```python
from build123d import *

# Parameters (mm, degrees)
BOSS_EXTRUDE1_DEPTH = 32
SKETCH2_R           = 5
CUT_EXTRUDE1_DEPTH  = 32


with BuildPart() as part:
    # Sketch1 → Boss-Extrude1 (new body)
    with BuildSketch(Plane.XY):
        with BuildLine():
            Line((-30, 0), (-13, 0))
            ThreePointArc((-13, 0), (0, -13), (13, 0))
            Line((13, 0), (30, 0))
            Line((30, 0), (30, -20))
            Line((30, -20), (-30, -20))
            Line((-30, -20), (-30, 0))
        make_face()
    extrude(amount=BOSS_EXTRUDE1_DEPTH)

    # Sketch2 → Cut-Extrude1 (cut)
    with BuildSketch(Plane.XZ.offset(20)):
        with Locations(Location((-19, 16, 0), (0, 0, 270))):
            Circle(SKETCH2_R)
        with Locations(Location((19, 16, 0), (0, 0, 270))):
            Circle(SKETCH2_R)
    extrude(amount=-CUT_EXTRUDE1_DEPTH, mode=Mode.SUBTRACT)


solid = part.part
```
Geometry check sheet. Reference: the model listing, model coordinates, mm. Give positions to 0.01 mm unless a question says otherwise; leave off trailing zeros. Write each loop counter-clockwise with the first axis right and the second up, starting at its lowest first coordinate (ties: lowest second). Pieces come first, ordered by that corner, then holes. Notation, with made-up numbers: (31, 12) -> (38, 12) arc R31 cw to (38, 50) -> close; hole circle Ø9 at (40.25, 41.5). An arc over 180 degrees is marked (long way). Use one line per item in the form item = value.
Item 1: Sectioned sample at C-C on z = 16. Enter the section's corners in (x, y), plus the area to 3 significant figures.
Results list:
outline = (-30, -20) -> (-24, -20) -> (-24, 0) -> (-30, 0) -> close; (-14, -20) -> (14, -20) -> (14, 0) -> (13, 0) arc R13 cw to (-13, 0) -> (-14, 0) -> close; (24, -20) -> (30, -20) -> (30, 0) -> (24, 0) -> close
area = 535 mm2
Item 2: Scan lines: line 1 (X direction, y = -14, z = 16); line 2 (X direction, y = -5.25, z = 16); line 3 (X direction, y = -6.25, z = 16). Record each from-to range of solid material in increasing order.
Results list:
line_1 = -30 to -24, -14 to 14, 24 to 30
line_2 = -30 to -24, -14 to -11.89, 11.89 to 14, 24 to 30
line_3 = -30 to -24, -14 to -11.4, 11.4 to 14, 24 to 30
Item 3: Sectioned sample at D-D on y = -5.75. Enter the section's corners in (x, z).
Results list:
outline = (-30, 0) -> (-11.66, 0) -> (-11.66, 32) -> (-30, 32) -> close; (11.66, 0) -> (30, 0) -> (30, 32) -> (11.66, 32) -> close; hole circle Ø10 at (-19, 16); hole circle Ø10 at (19, 16)
Item 4: Mould release check, pull along Z, two halves, no side actions. Record for faces 1 (the flat face through (25, 0, 16)), 2 (the flat face through (0, -14, 0)), 3 (the cylindrical face through (14.12, -10.14, 17.08)), 4 (the flat face through (0, -14, 32)): released by +Z, released by -Z, zero draft, split by the parting line, or undercut.
Results list:
face_1 = zero draft
face_2 = released by -Z
face_3 = undercut
face_4 = released by +Z
Item 5: Depth check by flat-ended pin: pin 1 Ø1.5 at (x, z) = (22.5, 17) entering from -Y. Enter the tip coordinate at first touch or a pass-through.
Results list:
pin_1 = through
Item 6: Sectioned sample at B-B on x = 19. Enter the section's corners in (y, z), plus the area to 3 significant figures.
Results list:
outline = (-20, 0) -> (0, 0) -> (0, 11) -> (-20, 11) -> close; (-20, 21) -> (0, 21) -> (0, 32) -> (-20, 32) -> close
area = 440 mm2
Item 7: Sectioned sample at A-A on y = -12. Enter the section's corners in (x, z).
Results list:
outline = (-30, 0) -> (-5, 0) -> (-5, 32) -> (-30, 32) -> close; (5, 0) -> (30, 0) -> (30, 32) -> (5, 32) -> close; hole circle Ø10 at (-19, 16); hole circle Ø10 at (19, 16)
